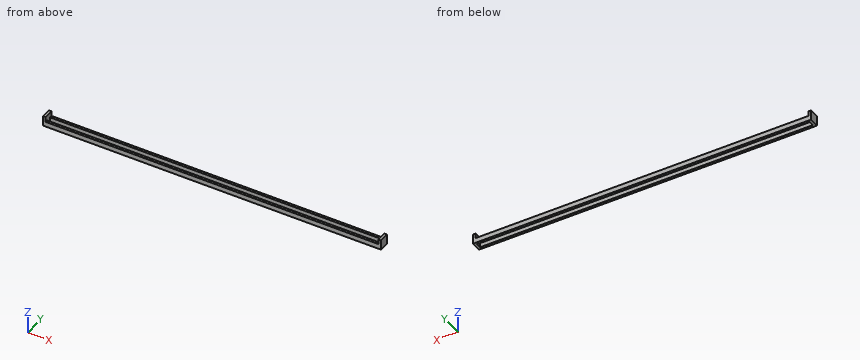
```python
from build123d import *

# Parameters (mm, degrees)
F0_W     = 215.9
F0_H     = 6.35
F0_W_2   = 212.725
F0_H_2   = 3.175
F1_DEPTH = 3.175
F3_DEPTH = 3.175


# Not quite as in the source:
# - a length typed as a fraction of an inch, garbled in the dataset ("3 / 203.2 mm" for 3/8 in), is restored


with BuildPart() as f1:
    # F0 (on Top) → F1 (new body)
    with BuildSketch(Plane.XY):
        with Locations((107.95, 3.175)):
            Rectangle(F0_W, F0_H)
        with Locations((107.95, 3.175)):
            Rectangle(F0_W_2, F0_H_2, mode=Mode.SUBTRACT)
    extrude(amount=F1_DEPTH)

    # F2 (on face) → F3 (join)
    with BuildSketch(Plane.XY.offset(3.175)):
        Polygon((1.5875, 0), (1.5875, 1.5875), (1.5875, 4.7625), (1.5875, 6.35), (0, 6.35), (0, 0), align=None)
        Polygon((214.3125, 4.7625), (214.3125, 1.5875), (214.3125, 0), (215.9, 0), (215.9, 6.35), (214.3125, 6.35), align=None)
    extrude(amount=F3_DEPTH)


solid = f1.part
```
The listing builds one solid part. Answer for the finished solid, in the listing's coordinates (mm). Give positions to 0.01 mm unless a question says otherwise; leave off trailing zeros. Order: outer loops, then holes, each group sorted by start corner. A loop starts at its lowest first (then second) coordinate and runs counter-clockwise, first axis right, second up. Notation, with made-up numbers: (8.5, -28) - (20.5, -28) arc R22 ccw to (20.5, 8) - close; hole circle Ø6 at (49.5, -35). An arc over 180 degrees is marked (long way). Answer in a Markdown table with one row per item. Add a question column.
Q1. Find the intervals of material crossed by line 1 along X through (y, z) = (3, 3.5); line 2 along Y through (x, z) = (72, 2.5); line 3 along Z through (x, y) = (104, 5.5) (3 decimals), in increasing order. Write a range as [from, to].
Q2. Given P1, Ø0.8, axis at x = 97, y = 6, coming from the +Z side (3 decimals), flat-ended and moving along its own axis, determine where the tip first touches the part or whether it passes through.
Q3. The part is cut by section A-A (y = 2.75). Determine the outline of the cut face in (x, z).
Determined:
| question | item | result |
|---|---|---|
| 1 | line 1 | x = [0, 1.59], [214.31, 215.9] |
| 1 | line 2 | y = [0, 1.59], [4.76, 6.35] |
| 1 | line 3 | z = [0, 3.175] |
| 2 | P1 | stops at z = 3.175 |
| 3 | outline | (0, 0) - (1.59, 0) - (1.59, 6.35) - (0, 6.35) - close; (214.31, 0) - (215.9, 0) - (215.9, 6.35) - (214.31, 6.35) - close |
